from build123d import *

# Parameters (mm, degrees)
F4_DEPTH = 5.08
F5_T     = -1.27
F3_R     = 1.524
F6_DEPTH = 25.4
F7_R     = 1.905
F8_DEPTH = 9.906
F9_R     = 2.54


with BuildPart() as f4:
    # F1 (on Top) → F4 (new body)
    with BuildSketch(Plane.XY):
        with BuildLine():
            ThreePointArc((21.59, 7.62), (20.102102, 11.212102), (16.51, 12.7))
            Line((16.51, 12.7), (-16.51, 12.7))
            ThreePointArc((-16.51, 12.7), (-20.102102, 11.212102), (-21.59, 7.62))
            Line((-21.59, 7.62), (-21.59, -7.62))
            ThreePointArc((-21.59, -7.62), (-20.102102, -11.212102), (-16.51, -12.7))
            Line((-16.51, -12.7), (16.51, -12.7))
            ThreePointArc((16.51, -12.7), (20.102102, -11.212102), (21.59, -7.62))
            Line((21.59, -7.62), (21.59, 7.62))
        make_face()
    extrude(amount=-F4_DEPTH)

    # F5
    f5_openings = [f4.faces().sort_by_distance(p)[0] for p in [
        (0, 0, 0),
    ]]
    offset(amount=F5_T, openings=f5_openings)

    # F3 (on offset) → F6 (cut)
    with BuildSketch(Plane.XY.offset(-7.62)):
        with Locations((15.24, -7.62)):
            Circle(F3_R)
        with Locations((15.24, 7.62)):
            Circle(F3_R)
        with Locations((5.08, -7.62)):
            Circle(F3_R)
        with Locations((-5.08, -7.62)):
            Circle(F3_R)
        with Locations((-15.24, -7.62)):
            Circle(F3_R)
        with Locations((5.08, 7.62)):
            Circle(F3_R)
        with Locations((-5.08, 7.62)):
            Circle(F3_R)
        with Locations((-15.24, 7.62)):
            Circle(F3_R)
    extrude(amount=-F6_DEPTH, mode=Mode.SUBTRACT)

    # F7 (on face) → F8 (cut)
    with BuildSketch(Plane.XY):
        with Locations((15.24, -7.62)):
            Circle(F7_R)
        with Locations((5.08, -7.62)):
            Circle(F7_R)
        with Locations((-5.08, -7.62)):
            Circle(F7_R)
        with Locations((-15.24, -7.62)):
            Circle(F7_R)
        with Locations((15.24, 7.62)):
            Circle(F7_R)
        with Locations((5.08, 7.62)):
            Circle(F7_R)
        with Locations((-5.08, 7.62)):
            Circle(F7_R)
        with Locations((-15.24, 7.62)):
            Circle(F7_R)
    extrude(amount=-F8_DEPTH, mode=Mode.SUBTRACT)

    # F9
    f9_edges = [f4.edges().sort_by_distance(p)[0] for p in [
        (0, -12.7, -5.08),
    ]]
    fillet(f9_edges, radius=F9_R)


solid = f4.part
Check sheet for the modelled part. Datum: model origin and axes. Units: mm. A direction names the side the tool comes from. Round coordinates to 2 decimals unless told otherwise and drop trailing zeros. Loops run counter-clockwise (first coordinate to the right, second up) from the corner with the lowest first, then second, coordinate; pieces in that order, holes last. Notation, with made-up numbers: (63, 78) -> (93, 78) arc R24 ccw to (93, 89) -> close; hole circle Ø11 at (82.25, -34.75). An arc over 180 degrees is marked (long way). Put each result on its own line as item: value. Start each with the question number.
1. Section check A-A (x = 15.24). Enter the section's corners in (y, z) (3 decimals).
2. Section check D-D (x = 0). Enter the section's corners in (y, z).
3. Section check C-C (y = 2.75). Enter the section's corners in (x, z).
4. Scan lines: probe 1 along Y at (x, z) = (6, -0.95); probe 2 along Y at (x, z) = (-15.24, -4.45) (3 decimals); probe 3 along Y at (x, z) = (-15.24, -4.15) (3 decimals). Record each from-to range of solid material in increasing order.
5. Draft check along Y on faces 1 (the face through (0, -12.7, -1)), 2 (the face through (0, 12.7, -1)), 3 (the face through (3.177, -7.536, -4.436)). Enter one of: +Y half, -Y half, draft (parallel to the pull), parting line (faces both ways), or undercut.
6. Access from +Z, -Z, +X, -X, +Y, -Y to the whole of each face (thin tool, end or side, straight path). Record for faces 4 (the face through (-19.234, -10.284, -1.878)), 5 (the face through (20.141, 11.172, -1.252)).
7. Section check B-B (z = -3.4). Enter the section's corners in (x, y).
8. Gauge pin test, flat ends, axial feed: pin 1 (3.5 mm diameter, centred on x = -15.24, y = 7.62, fed in from -Z); pin 2 (6 mm diameter, centred on x = 15.24, y = 7.62, fed in from +Z); pin 3 (1.5 mm diameter, centred on x = 15, z = -4, fed in from +Y). Record the tip position at first contact, or that the pin passes through.
Findings:
1. outline: (-12.7, -2.54) arc R2.54 ccw to (-10.16, -5.08) -> (-9.525, -5.08) -> (-9.525, -3.81) -> (-11.43, -3.81) -> (-11.43, 0) -> (-12.7, 0) -> close; (-5.715, -5.08) -> (5.715, -5.08) -> (5.715, -3.81) -> (-5.715, -3.81) -> close; (9.525, -5.08) -> (10.16, -5.08) arc R2.54 ccw to (12.7, -2.54) -> (12.7, 0) -> (11.43, 0) -> (11.43, -3.81) -> (9.525, -3.81) -> close
2. outline: (-12.7, -2.54) arc R2.54 ccw to (-10.16, -5.08) -> (10.16, -5.08) arc R2.54 ccw to (12.7, -2.54) -> (12.7, 0) -> (11.43, 0) -> (11.43, -3.81) -> (-11.43, -3.81) -> (-11.43, 0) -> (-12.7, 0) -> close
3. outline: (-21.59, -2.54) arc R2.54 ccw to (-19.05, -5.08) -> (19.05, -5.08) arc R2.54 ccw to (21.59, -2.54) -> (21.59, 0) -> (20.32, 0) -> (20.32, -3.81) -> (-20.32, -3.81) -> (-20.32, 0) -> (-21.59, 0) -> close
4. probe 1: y = -12.7 to -11.43, 11.43 to 12.7
4. probe 2: y = -11.834 to -9.525, -5.715 to 5.715, 9.525 to 11.834
4. probe 3: y = -12.125 to -9.525, -5.715 to 5.715, 9.525 to 12.125
5. face 1: -Y half
5. face 2: +Y half
5. face 3: undercut
6. face 4: +Z
6. face 5: +Z, -Z, +X, +Y
7. outline: (-21.44, -7.62) arc R4.93 ccw to (-16.51, -12.55) -> (16.51, -12.55) arc R4.93 ccw to (21.44, -7.62) -> (21.44, 7.62) arc R4.93 ccw to (16.51, 12.55) -> (-16.51, 12.55) arc R4.93 ccw to (-21.44, 7.62) -> close; hole (-20.32, -7.62) arc R3.81 ccw to (-16.51, -11.43) -> (16.51, -11.43) arc R3.81 ccw to (20.32, -7.62) -> (20.32, 7.62) arc R3.81 ccw to (16.51, 11.43) -> (-16.51, 11.43) arc R3.81 ccw to (-20.32, 7.62) -> close
8. pin 1: passes through
8. pin 2: stops at z = -3.81
8. pin 3: stops at y = 12.6
